Can you work these out from the model? Positions are in its coordinate system, mm. A direction names the side the tool comes from. Round coordinates to 2 decimals unless told otherwise and drop trailing zeros. Loops run counter-clockwise (first coordinate to the right, second up) from the corner with the lowest first, then second, coordinate; pieces in that order, holes last. Notation, with made-up numbers: (39.25, 38) -> (70.25, 38) arc R20 cw to (70.25, 58) -> close; hole circle Ø2 at (50, 8.5). An arc over 180 degrees is marked (long way). Write item = value, one per line.
from build123d import *

# Parameters (mm, degrees)
F0_W     = 31
F0_H     = 22
F0_W_2   = 27
F0_H_2   = 18
F1_DEPTH = 45
F2_R     = 2
F3_R     = 1.5


with BuildPart() as f1:
    # F0 (on Front) → F1 (new body)
    with BuildSketch(Plane.XZ):
        with Locations((13.5, 9)):
            Rectangle(F0_W, F0_H)
        with Locations((13.5, 9)):
            Rectangle(F0_W_2, F0_H_2, mode=Mode.SUBTRACT)
    extrude(amount=F1_DEPTH)

    # F2
    f2_edges = [f1.edges().sort_by_distance(p)[0] for p in [
        (29, -22.5, 20),
        (-2, -22.5, 20),
        (29, -22.5, -2),
        (-2, -22.5, -2),
    ]]
    fillet(f2_edges, radius=F2_R)

    # F3
    f3_edges = [f1.edges().sort_by_distance(p)[0] for p in [
        (27, -22.5, 18),
        (27, -22.5, 0),
        (0, -22.5, 0),
        (0, -22.5, 18),
    ]]
    fillet(f3_edges, radius=F3_R)


solid = f1.part
1. Suppose I cut it at B-B, the plane z = 7.75. List the corners of the cut face in (x, y) for me.
Entries:
outline = (-2, -45) -> (0, -45) -> (0, 0) -> (-2, 0) -> close; (27, -45) -> (29, -45) -> (29, 0) -> (27, 0) -> close
2. I need wall thicknesses on line 1 (Z direction, x = 23, y = -31.5); line 2 (X direction, y = -14.5, z = 4); line 3 (X direction, y = -36.5, z = -1). Which ranges of each line are inside material? Lowest first, please. Write a range as [from, to].
Entries:
line_1 = [-2, 0], [18, 20]
line_2 = [-2, 0], [27, 29]
line_3 = [-1.73, 28.73]
3. For faces 1 (the cylindrical face through (-1.43, -22.82, 19.4)), 2 (the cylindrical face through (0.45, -22.82, 0.43)), which set-ups out of +Z, -Z, +X, -X, +Y, -Y let a thin tool reach every point of the face, with its end or its side?
Entries:
face_1 = +Z, -X, +Y, -Y
face_2 = +Y, -Y
4. Suppose I cut it at C-C, the plane y = -38.5. List the corners of the cut face in (x, z) for me.
Entries:
outline = (-2, 0) arc R2 ccw to (0, -2) -> (27, -2) arc R2 ccw to (29, 0) -> (29, 18) arc R2 ccw to (27, 20) -> (0, 20) arc R2 ccw to (-2, 18) -> close; hole (0, 1.5) arc R1.5 ccw to (1.5, 0) -> (25.5, 0) arc R1.5 ccw to (27, 1.5) -> (27, 16.5) arc R1.5 ccw to (25.5, 18) -> (1.5, 18) arc R1.5 ccw to (0, 16.5) -> close
5. Suppose I cut it at A-A, the plane x = 2.5. List the corners of the cut face in (y, z) for me.
Entries:
outline = (-45, -2) -> (0, -2) -> (0, 0) -> (-45, 0) -> close; (-45, 18) -> (0, 18) -> (0, 20) -> (-45, 20) -> close
